CAD build for the part. Positions are in the model's coordinates, mm. Give positions to 0.01 mm unless a question says otherwise; leave off trailing zeros. Write each loop counter-clockwise with the first axis right and the second up, starting at its lowest first coordinate (ties: lowest second). Pieces come first, ordered by that corner, then holes. Notation, with made-up numbers: (31, 12.25) -> (47, 12.25) arc R14 ccw to (47, 37.25) -> close; hole circle Ø10 at (60.5, -37.5). An arc over 180 degrees is marked (long way). Use one line per item in the form item = value. Start each with the question number.
from build123d import *

# Parameters (mm, degrees)
SKETCH1_R           = 1.55
SKETCH1_R_2         = 1.5
BOSS_EXTRUDE1_DEPTH = 2


with BuildPart() as part:
    # Sketch1 → Boss-Extrude1 (new body)
    with BuildSketch(Plane.XY):
        Polygon((0, 20.8), (8.5, 20.8), (8.5, 37.6), (0, 37.6), (0, 56.6), (8.5, 56.6), (8.5, 73.4), (0, 73.4), (0, 92.4), (8.5, 92.4), (8.5, 109.2), (0, 109.2), (0, 128.2), (8.5, 128.2), (8.5, 145), (0, 145), (0, 164), (8.5, 164), (8.5, 173), (263.5, 173), (263.5, 164), (272, 164), (272, 145), (263.5, 145), (263.5, 128.2), (272, 128.2), (272, 109.2), (263.5, 109.2), (263.5, 92.4), (272, 92.4), (272, 73.4), (263.5, 73.4), (263.5, 56.6), (272, 56.6), (272, 37.6), (263.5, 37.6), (263.5, 20.8), (272, 20.8), (272, 0), (0, 0), align=None)
        with Locations((4.25, 154.5)):
            Circle(SKETCH1_R, mode=Mode.SUBTRACT)
        with Locations((4.25, 118.5)):
            Circle(SKETCH1_R, mode=Mode.SUBTRACT)
        with Locations((4.25, 82.5)):
            Circle(SKETCH1_R, mode=Mode.SUBTRACT)
        with Locations((4.25, 46.5)):
            Circle(SKETCH1_R, mode=Mode.SUBTRACT)
        with Locations((4.25, 10.5)):
            Circle(SKETCH1_R, mode=Mode.SUBTRACT)
        with Locations(Location((267.75, 10.5, 0), (0, 0, 180))):
            Circle(SKETCH1_R, mode=Mode.SUBTRACT)
        with Locations(Location((267.75, 46.5, 0), (0, 0, 180))):
            Circle(SKETCH1_R, mode=Mode.SUBTRACT)
        with Locations(Location((267.75, 82.5, 0), (0, 0, 180))):
            Circle(SKETCH1_R, mode=Mode.SUBTRACT)
        with Locations(Location((267.75, 118.5, 0), (0, 0, 180))):
            Circle(SKETCH1_R, mode=Mode.SUBTRACT)
        with Locations(Location((267.75, 154.5, 0), (0, 0, 180))):
            Circle(SKETCH1_R, mode=Mode.SUBTRACT)
        with Locations((25.5, 11.75)):
            Circle(SKETCH1_R_2, mode=Mode.SUBTRACT)
        with Locations((136, 11.75)):
            Circle(SKETCH1_R_2, mode=Mode.SUBTRACT)
        with Locations((246.5, 11.75)):
            Circle(SKETCH1_R_2, mode=Mode.SUBTRACT)
    extrude(amount=BOSS_EXTRUDE1_DEPTH)


solid = part.part
1) Pin check, flat tip, straight feed: pin 1 (1 mm diameter, centred on x = 3.5, z = 1.5, fed in from +Y). Stop position of the tip, or through.
2) Wall check: line 1 along X through (y, z) = (82.5, 1.4); line 2 along Y through (x, z) = (136, 1.55); line 3 along X through (y, z) = (61.5, 0.8). Give the ranges that are in metal, low to high. Write a range as from..to.
3) Cut at B-B (y = 104). Give the cut face in (x, z), and give its area (3 significant figures).
4) Cut at A-A (z = 1). State how many separate pieces and enclosed holes the cut face has, and give its area (3 significant figures).
Final values:
q1.pin_1 = 164
q2.line_1 = 0..2.7, 5.8..266.2, 269.3..272
q2.line_2 = 0..10.25, 13.25..173
q2.line_3 = 8.5..263.5
q3.outline = (8.5, 0) -> (263.5, 0) -> (263.5, 2) -> (8.5, 2) -> close
q3.area = 510 mm^2
q4.separate_pieces = 1
q4.enclosed_holes = 13
q4.area = 45,700 mm^2
